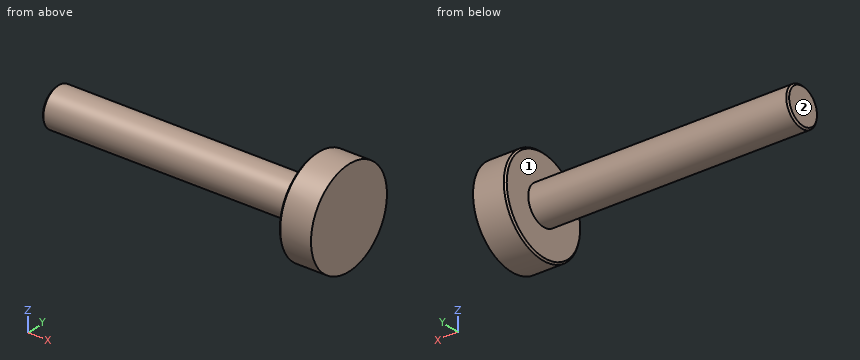
from build123d import *

# Parameters (mm, degrees)
F0_R     = 15
F1_DEPTH = 10
F2_R     = 6
F3_DEPTH = 80
F4_SIZE  = 0.5


with BuildPart() as f1:
    # F0 (on Right) → F1 (new body)
    with BuildSketch(Plane.YZ):
        Circle(F0_R)
    extrude(amount=-F1_DEPTH)

    # F2 (on face) → F3 (join)
    with BuildSketch(Plane(origin=(-10, 0, 0), x_dir=(0, -1, 0), z_dir=(-1, 0, 0))):
        Circle(F2_R)
    extrude(amount=F3_DEPTH)

    # F4
    f4_edges = [f1.edges().sort_by_distance(p)[0] for p in [
        (-90, 6, 0),
        (-10, -15, 0),
    ]]
    chamfer(f4_edges, length=F4_SIZE)


solid = f1.part
CAD build for the part. Positions are in the model's coordinates, mm. Face numbers are marked on the shaded views. A direction names the side the tool comes from. Give positions to 0.01 mm unless a question says otherwise; leave off trailing zeros. Loops run counter-clockwise (first coordinate to the right, second up) from the corner with the lowest first, then second, coordinate; pieces in that order, holes last. Notation, with made-up numbers: M -5.75,74.5 L 48.25,74.5 A20 ccw 48.25,101.5 Z; hole C 12.25,21 d8. An arc over 180 degrees is marked long. One line per question, with ' | ' between items. Start each with the question number.
1. 3-axis set-ups, long thin cutter, end or side, ignore diameter. For the marked faces 1 and 2: which of +Z, -Z, +X, -X, +Y, -Y reach the whole face in a straight line?
2. Flat gauge pins, fed straight in: pin 1 (8 mm diameter, centred on y = 4.5, z = 10.5, fed in from -X); pin 2 (12 mm diameter, centred on x = -28.5, y = -5, fed in from +Z); pin 3 (2 mm diameter, centred on x = -15, z = 2, fed in from +Y); pin 4 (3 mm diameter, centred on x = -48, y = 9, fed in from -Z). Where does each tip first touch, or does it go through?
3. Saw through at A-A on y = 0. Give the cut face in (x, z), plus the area to 3 significant figures.
4. Probe L1, parallel to X at y = -13, z = 2; L2, parallel to Y at x = -31, z = 0.25; L3, parallel to Z at x = -31, y = -0.5. List the from-to ranges inside material, lowest first. Write a range as from..to.
5. Saw through at C-C on x = -73.5. Give the cut face in (y, z), plus the area to 3 significant figures.
Result sheet:
1) face 1: -X | face 2: +Z, -Z, -X, +Y, -Y
2) pin 1: stops at x = -10 | pin 2: stops at z = 6 | pin 3: stops at y = 5.92 | pin 4: passes through
3) outline: M -90,-5.5 L -89.5,-6 L -10,-6 L -10,-14.5 L -9.5,-15 L 0,-15 L 0,15 L -9.5,15 L -10,14.5 L -10,6 L -89.5,6 L -90,5.5 Z | area: 1,260 mm^2
4) L1: x = -10..0 | L2: y = -5.99..5.99 | L3: z = -5.98..5.98
5) outline: C 0,0 d12 | area: 113 mm^2
